```python
from build123d import *

# Parameters (mm, degrees)
RECTWITHARC_W              = 275
RECTWITHARC_H              = 50
ARMBASE_DEPTH              = 50
CUT_EXTRUDE1_REACH         = 307.164
HOLLOWMIDDLE_DEPTH         = 15
HOLLOWMIDDLE_DEPTH_BACK    = 306.163890393
SKETCH1_W                  = 210
SKETCH1_H                  = 30
JOINT2SHAFTHOLE_DEPTH      = 306.163890393
JOINT2SHAFTHOLE_DEPTH_BACK = 10
J2SHAFTCOUNTERSINK_START   = 50
SKETCH4_R                  = 20
J2SHAFTCOUNTERSINK_DEPTH   = 10
HOLDINGHOLE_START          = 15
HOLDINGHOLE_OUTLINE_R      = 5
HOLDINGHOLE_DEPTH          = 10
COUNTERSINK_R              = 7.5
COUNTERSINKCUT_DEPTH       = 1
MOUNTING_START             = 235
SKETCH6_R                  = 7
MOUNTING_HOLE_DEPTH        = 30
COUNTERSINK2_START         = 235
SKETCH7_R                  = 9
COUNTERSINK2_DEPTH         = 3
SKETCH8_R                  = 27.5
ARMCUTOUT_DEPTH            = 30


# Read off the part's stored shape, not the designer's step: HoldingHole
with BuildPart() as part:
    # RectwithArc → ArmBase (new body)
    with BuildSketch(Plane(origin=(0, 0, 0), x_dir=(1, 0, 0), z_dir=(0, 1, 0))):
        with BuildLine():
            ThreePointArc((0, -25), (-25, 0), (0, 25))
            Line((0, 25), (0, -25))
        make_face()
        with Locations((137.5, 0)):
            Rectangle(RECTWITHARC_W, RECTWITHARC_H)
        with BuildLine():
            Line((275, 25), (275, -25))
            ThreePointArc((275, -25), (300, 0), (275, 25))
        make_face()
    extrude(amount=ARMBASE_DEPTH)

    # ShaftKey → Cut-Extrude1 (cut, up to next)
    with BuildSketch(Plane(origin=(0, 0, 0), x_dir=(1, 0, 0), z_dir=(0, 1, 0)), mode=Mode.PRIVATE) as cut_extrude1_sk1:
        with BuildLine():
            Line((15, 9.013878189), (15, -9.013878189))
            ThreePointArc((15, -9.013878189), (-17.5, 0), (15, 9.013878189))
        make_face()
    cut_extrude1_tool1 = extrude(cut_extrude1_sk1.sketch, amount=CUT_EXTRUDE1_REACH, mode=Mode.PRIVATE) & part.part
    add(cut_extrude1_tool1.solids().sort_by_distance((-0.524095, 0, 0))[0], mode=Mode.SUBTRACT)

    # Sketch1 → HollowMIddle (cut, two sides: drawn at the far end of the back side and taken through both)
    with BuildSketch(Plane.XY.offset(-HOLLOWMIDDLE_DEPTH_BACK)):
        with Locations((130, 25)):
            Rectangle(SKETCH1_W, SKETCH1_H)
    extrude(amount=HOLLOWMIDDLE_DEPTH + HOLLOWMIDDLE_DEPTH_BACK, mode=Mode.SUBTRACT)

    # J2ShaftHole → Joint2ShaftHole (cut, two sides: drawn at the far end of the back side and taken through both)
    with BuildSketch(Plane(origin=(0, 0, 0), x_dir=(1, 0, 0), z_dir=(0, 1, 0)).offset(-JOINT2SHAFTHOLE_DEPTH_BACK)):
        with BuildLine():
            Line((265, 11.180339887), (265, -11.180339887))
            ThreePointArc((265, -11.180339887), (290, 0), (265, 11.180339887))
        make_face()
    extrude(amount=JOINT2SHAFTHOLE_DEPTH + JOINT2SHAFTHOLE_DEPTH_BACK, mode=Mode.SUBTRACT)

    # Sketch4 → J2ShaftCounterSink (cut)
    with BuildSketch(Plane(origin=(0, 0, 0), x_dir=(1, 0, 0), z_dir=(0, 1, 0)).offset(J2SHAFTCOUNTERSINK_START)):
        with Locations(Location((275, 0, 0), (0, 0, 270))):
            Circle(SKETCH4_R)
    extrude(amount=-J2SHAFTCOUNTERSINK_DEPTH, mode=Mode.SUBTRACT)

    # HoldingHole outline → HoldingHole (cut)
    with BuildSketch(Plane(origin=(0, 0, 0), x_dir=(0, 0, -1), z_dir=(1, 0, 0)).offset(HOLDINGHOLE_START)):
        with Locations((0, 24)):
            Circle(HOLDINGHOLE_OUTLINE_R)
    extrude(amount=HOLDINGHOLE_DEPTH, mode=Mode.SUBTRACT)

    # CounterSink → CounterSinkCut (cut)
    with BuildSketch(Plane(origin=(25, 0, 0), x_dir=(0, 0, -1), z_dir=(1, 0, 0))):
        with Locations(Location((0, 24, 0), (0, 0, 90))):
            Circle(COUNTERSINK_R)
    extrude(amount=-COUNTERSINKCUT_DEPTH, mode=Mode.SUBTRACT)

    # Sketch6 → Mounting Hole (cut)
    with BuildSketch(Plane(origin=(0, 0, 0), x_dir=(0, 0, -1), z_dir=(1, 0, 0)).offset(MOUNTING_START)):
        with Locations((0, 25)):
            Circle(SKETCH6_R)
    extrude(amount=MOUNTING_HOLE_DEPTH, mode=Mode.SUBTRACT)

    # Sketch7 → CounterSink2 (cut)
    with BuildSketch(Plane(origin=(0, 0, 0), x_dir=(0, 0, -1), z_dir=(1, 0, 0)).offset(COUNTERSINK2_START)):
        with Locations((0, 25)):
            Circle(SKETCH7_R)
    extrude(amount=COUNTERSINK2_DEPTH, mode=Mode.SUBTRACT)

    # Sketch8 → ArmCutout (cut)
    with BuildSketch(Plane(origin=(0, 0, 0), x_dir=(1, 0, 0), z_dir=(0, 1, 0))):
        with Locations((275, 0)):
            Circle(SKETCH8_R)
    extrude(amount=ARMCUTOUT_DEPTH, mode=Mode.SUBTRACT)


solid = part.part
```
Here's how the part is built. I have some questions about the finished solid (model axes, mm). A direction names the side the tool comes from. Give positions to 0.01 mm unless a question says otherwise; leave off trailing zeros. Loops run counter-clockwise (first coordinate to the right, second up) from the corner with the lowest first, then second, coordinate; pieces in that order, holes last. Notation, with made-up numbers: M 69.5,-29 L 77.5,-29 A21 cw 77.5,10 Z; hole C 15.25,45 d5. An arc over 180 degrees is marked long. Use one line per item in the form item = value. Start each with the question number.
Q1. If we section it at B-B (x = 171): Write out the boundary of the cut face in (y, z).
Q2. If we section it at C-C (z = 0): State how many separate pieces and enclosed holes the cut face has, then the cut area to 3 significant figures.
Q3. If we section it at A-A (y = 3.5): Write out the boundary of the cut face in (x, z).
Q4. Will these pins go through, and if not, where does the flat tip stop? pin 1 Ø6 at (y, z) = (13.5, 4.5) entering from -X; pin 2 Ø9 at (y, z) = (24, 0) entering from +X; pin 3 Ø3 at (y, z) = (17, 9) entering from -X.
Q5. I need wall thicknesses on line 1 along Y through (x, z) = (76, 13.5); line 2 along Z through (x, y) = (275, 34.5); line 3 along X through (y, z) = (20.5, -10). Which ranges of each line are inside material? Lowest first, please.
Q6. Thinking about a two-plate mould opening in X: for faces 1 (the cylindrical face through (299.994, 39.86, 0.55)), 2 (the flat face through (136, 41, -25)), 3 (the cylindrical face through (-17.49, 24.65, 0.64)), which applies, +X half, -X half, draft (parallel to the pull), parting line (faces both ways), or undercut?
Q7. Which directions (+Z, -Z, +X, -X, +Y, -Y) give clear straight access to the entire face, cutting with the end or side of a thin tool? Please do faces 4 (the flat face through (24, 29, -2)), 5 (the cylindrical face through (19.44, 19.12, 1.08)), 6 (the flat face through (262, 40, 0)), 7 (the flat face through (25, 25, -10)).
Taken from the geometry:
q1.outline = M 0,-25 L 10,-25 L 10,15 L 40,15 L 40,-25 L 50,-25 L 50,25 L 0,25 Z
q2.separate_pieces = 4
q2.enclosed_holes = 0
q2.area = 5,770 mm^2
q3.outline = M 0,-25 L 263.54,-25 A27.5 cw 263.54,25 L 0,25 A25 ccw Z; hole M 15,-9.01 L 15,9.01 A17.5 ccw long Z
q4.pin_1 = -24.95
q4.pin_2 = -16.91
q4.pin_3 = -23.85
q5.line_1 = 0 to 10, 40 to 50
q5.line_2 = -25 to -15, 15 to 25
q5.line_3 = -22.91 to -14.36, 14.36 to 25, 235 to 249.38
q6.face_1 = +X half
q6.face_2 = draft
q6.face_3 = undercut
q7.face_4 = none
q7.face_5 = +X
q7.face_6 = +Y
q7.face_7 = -Z
